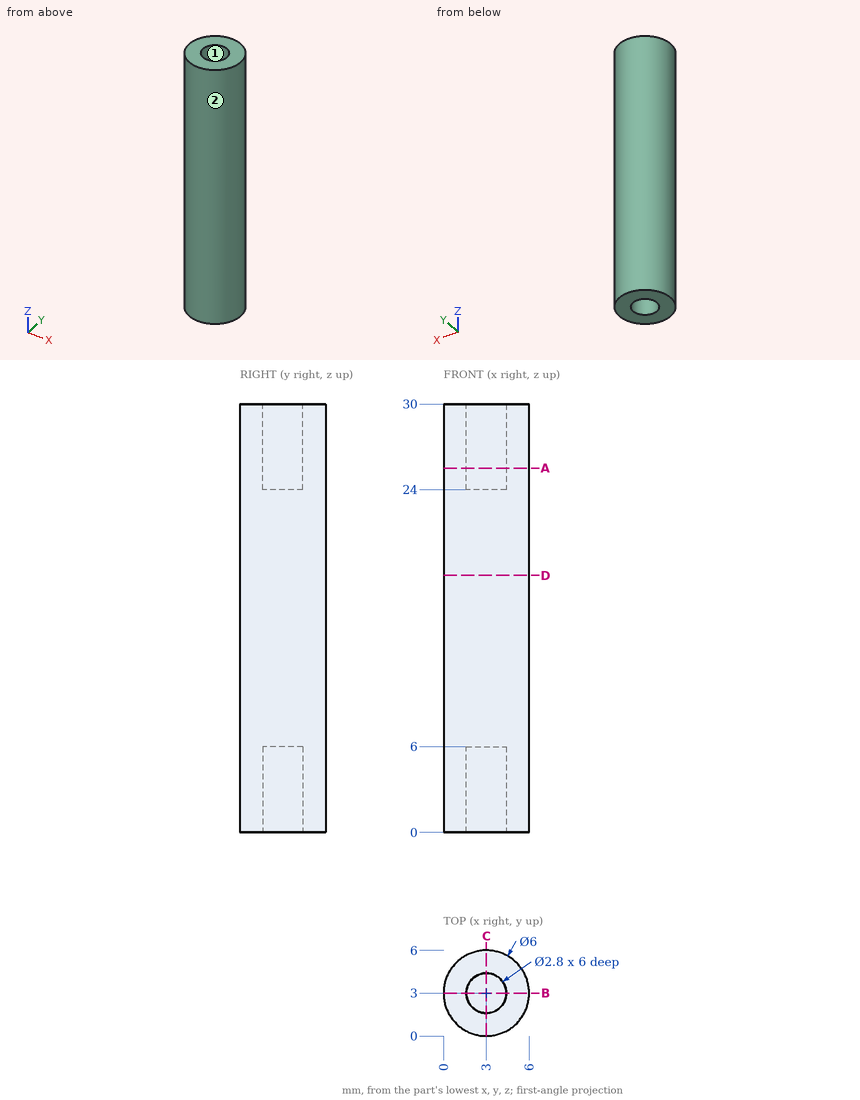
Check sheet for the drawn part. Datum: minimum x, y, z corner. Units: mm. Coordinates: 2 decimals unless noted, no trailing zeros. Loops run counter-clockwise (first coordinate to the right, second up) from the corner with the lowest first, then second, coordinate; pieces in that order, holes last. Notation, with made-up numbers: (23.5, 16) -> (77.5, 16) arc R35 ccw to (77.5, 51) -> close; hole circle Ø3 at (19, -3.5). An arc over 180 degrees is marked (long way). Answer as CSV lines item,"result".
1) Cross-section at D-D, the plane z = 18. Record the cut outline in (x, y).
Found:
outline,"circle Ø6 at (3, 3)"
2) Release check for a two-part mould opening along Y. For the marked faces 1 and 2 record: +Y half, -Y half, draft (parallel to the pull), parting line (faces both ways), or undercut.
Found:
face 1,"undercut"
face 2,"parting line"
3) Depth check by flat-ended pin: pin 1 (2.5 mm diameter, centred on x = 3, y = 3, fed in from -Z); pin 2 (1 mm diameter, centred on x = 5.5, z = 10.5, fed in from -Y); pin 3 (1.4 mm diameter, centred on x = 3, y = 3.5, fed in from +Z). Enter the tip coordinate at first touch or a pass-through.
Found:
pin 1,"stops at z = 6"
pin 2,"stops at y = 0.76"
pin 3,"stops at z = 24"
4) Thickness scan on L1, parallel to Y at x = 3, z = 27.85; L2, parallel to Y at x = 3.75, z = 25; L3, parallel to Z at x = 1.7, y = 2.9. Record the ranges inside material, lowest first. Write a range as from..to.
Found:
L1,"y = 0..1.6, 4.4..6"
L2,"y = 0.1..1.82, 4.18..5.9"
L3,"z = 6..24"
5) Cross-section at A-A, the plane z = 25.5. Record the cut outline in (x, y), then the cut area to 3 significant figures.
Found:
outline,"circle Ø6 at (3, 3); hole circle Ø2.8 at (3, 3)"
area,"22.1 mm2"
6) Cross-section at B-B, the plane y = 3. Record the cut outline in (x, z).
Found:
outline,"(0, 0) -> (1.6, 0) -> (1.6, 6) -> (4.4, 6) -> (4.4, 0) -> (6, 0) -> (6, 30) -> (4.4, 30) -> (4.4, 24) -> (1.6, 24) -> (1.6, 30) -> (0, 30) -> close"
